Work out the finished part from the listing and answer in its coordinate system (mm). Face numbers are marked on the shaded views. A direction names the side the tool comes from. Round coordinates to 2 decimals unless told otherwise and drop trailing zeros. Order: outer loops, then holes, each group sorted by start corner. A loop starts at its lowest first (then second) coordinate and runs counter-clockwise, first axis right, second up.
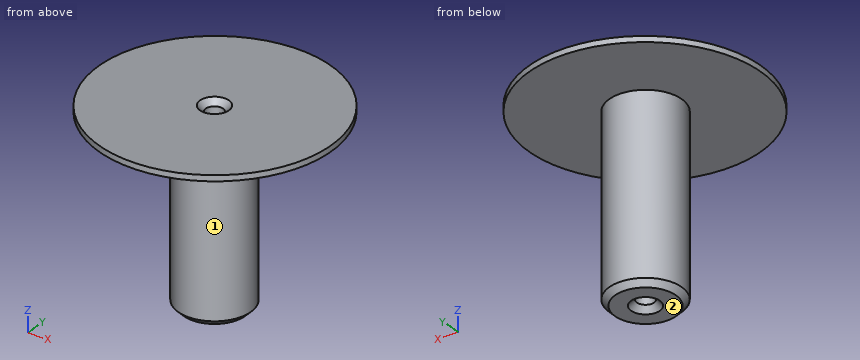
from build123d import *

# Parameters (mm, degrees)
SKETCH1_R           = 1.25
SKETCH1_R_2         = 0.3
BOSS_EXTRUDE1_DEPTH = 6.5
SKETCH2_R           = 4
SKETCH2_R_2         = 1.25
BOSS_EXTRUDE2_DEPTH = 0.2
CHAMFER1_SIZE       = 0.2


with BuildPart() as part:
    # Sketch1 → Boss-Extrude1 (new body)
    with BuildSketch(Plane.XY):
        Circle(SKETCH1_R)
        Circle(SKETCH1_R_2, mode=Mode.SUBTRACT)
    extrude(amount=BOSS_EXTRUDE1_DEPTH)

    # Sketch2 → Boss-Extrude2 (add)
    with BuildSketch(Plane.XY.offset(6.5)):
        with Locations((0.018669882, 0)):
            Circle(SKETCH2_R)
        Circle(SKETCH2_R_2, mode=Mode.SUBTRACT)
    extrude(amount=-BOSS_EXTRUDE2_DEPTH)

    # Chamfer1
    chamfer1_edges = [part.edges().sort_by_distance(p)[0] for p in [
        (-1.25, 0, 0),
        (-0.3, 0, 0),
        (-0.3, 0, 6.5),
    ]]
    chamfer(chamfer1_edges, length=CHAMFER1_SIZE)


solid = part.part
Item 1: Find the intervals of material crossed by line 1 along Y through (x, z) = (0, 1.75); line 2 along Z through (x, y) = (1.5, 0); line 3 along X through (y, z) = (-1, 4.25), in increasing order.
Item 2: Find section A-A (y = 0). Write down the section's boundary in (x, z), plus the area to 3 significant figures.
Item 3: Find section B-B (x = 0). Write down the section's boundary in (y, z), plus the area to 3 significant figures.
Item 4: A tool of negligible diameter and unlimited length cuts with its end or side. For the marked faces 1 and 2, from which of +Z, -Z, +X, -X, +Y, -Y can it reach the whole face along a straight path? Write none if from no direction.
Item 5: Given pin 1 (2 mm diameter, centred on y = 0, z = 3.5, fed in from +X); pin 2 (3 mm diameter, centred on y = -2.5, z = 1, fed in from -X); pin 3 (2 mm diameter, centred on x = 2, z = 5.5, fed in from -Y), each flat-ended and moving along its own axis, determine where each tip first touches the part or whether it passes through.
Item 6: Find section C-C (z = 0.75). Write down the section's boundary in (x, y), plus the area to 3 significant figures.
Item 7: Find section D-D (x = 3). Write down the section's boundary in (y, z), plus the area to 3 significant figures.
Model answer:
1. line 1: y = -1.25 to -0.3, 0.3 to 1.25
1. line 2: z = 6.3 to 6.5
1. line 3: x = -0.75 to 0.75
2. outline: (-3.98, 6.3) - (-1.25, 6.3) - (-1.25, 0.2) - (-1.05, 0) - (-0.5, 0) - (-0.3, 0.2) - (-0.3, 6.3) - (-0.5, 6.5) - (-3.98, 6.5) - close; (0.3, 0.2) - (0.5, 0) - (1.05, 0) - (1.25, 0.2) - (1.25, 6.3) - (4.02, 6.3) - (4.02, 6.5) - (0.5, 6.5) - (0.3, 6.3) - close
2. area: 13.3 mm2
3. outline: (-4, 6.3) - (-1.25, 6.3) - (-1.25, 0.2) - (-1.05, 0) - (-0.5, 0) - (-0.3, 0.2) - (-0.3, 6.3) - (-0.5, 6.5) - (-4, 6.5) - close; (0.3, 0.2) - (0.5, 0) - (1.05, 0) - (1.25, 0.2) - (1.25, 6.3) - (4, 6.3) - (4, 6.5) - (0.5, 6.5) - (0.3, 6.3) - close
3. area: 13.3 mm2
4. face 1: -Z
4. face 2: -Z, +X, -X, +Y, -Y
5. pin 1: stops at x = 1.25
5. pin 2: stops at x = -0.75
5. pin 3: stops at y = -3.75
6. outline: circle Ø2.5 at (0, 0); hole circle Ø0.6 at (0, 0)
6. area: 4.63 mm2
7. outline: (-2.67, 6.3) - (2.67, 6.3) - (2.67, 6.5) - (-2.67, 6.5) - close
7. area: 1.07 mm2
